from build123d import *

# Parameters (mm, degrees)
PAD_DEPTH           = 6
HOLE_D              = 6.6
HOLE_DEPTH          = 25
HOLE_CSINK_D        = 13.44
HOLE_CSINK_ANGLE    = 90
HOLE001_D           = 3.3
HOLE001_CSINK_D     = 4.05
HOLE001_CSINK_ANGLE = 90


with BuildPart() as part:
    # Sketch → Pad (new body)
    with BuildSketch(Plane.XY):
        with BuildLine():
            Line((0, 4.242641), (4.242641, 0))
            Line((177.999997, 0), (4.242641, 0))
            ThreePointArc((177.999997, 0), (179.414214, 0.585787), (180, 2.000004))
            Line((180, 161.757359), (180, 2.000004))
            Line((175.757359, 166), (180, 161.757359))
            Line((2.000009, 166), (175.757359, 166))
            ThreePointArc((2.000009, 166), (0.585793, 165.414221), (0, 164.000011))
            Line((0, 4.242641), (0, 164.000011))
        make_face()
    extrude(amount=PAD_DEPTH)

    # Hole
    with Locations(Plane.XY.offset(6)):
        with Locations((12, 154), (168, 154), (168, 12), (12, 12)):
            CounterSinkHole(HOLE_D / 2, HOLE_CSINK_D / 2, depth=HOLE_DEPTH, counter_sink_angle=HOLE_CSINK_ANGLE)

    # Hole001 (through all)
    with Locations(Plane.XY.offset(6)):
        with Locations((69.693453, 152.79207), (78.426115, 150.614773), (87.158776, 148.437476), (68, 146), (76.732662, 143.822703), (85.465323, 141.645406)):
            CounterSinkHole(HOLE001_D / 2, HOLE001_CSINK_D / 2, counter_sink_angle=HOLE001_CSINK_ANGLE)


solid = part.part
Geometry check sheet. Reference: the model listing, model coordinates, mm. Round coordinates to 2 decimals unless told otherwise and drop trailing zeros. Order: outer loops, then holes, each group sorted by start corner. A loop starts at its lowest first (then second) coordinate and runs counter-clockwise, first axis right, second up. Notation, with made-up numbers: (71, -40) - (91, -40) arc R27 cw to (91, -10) - close; hole circle Ø11 at (-4.75, 11.5). An arc over 180 degrees is marked (long way). One line per question, with ' | ' between items. Start each with the question number.
(1) Thickness scan on L1, parallel to Y at x = 168, z = 2.05; L2, parallel to X at y = 147, z = 1.65; L3, parallel to Y at x = 15, z = 5.1. Record the ranges inside material, lowest first. Write a range as [from, to].
(2) Sectioned sample at A-A on x = 12. Record the cut outline in (y, z), and give its area (3 significant figures).
(3) Sectioned sample at B-B on y = 12. Record the cut outline in (x, z).
(4) Depth check by flat-ended pin: pin 1 Ø6 at (x, y) = (12, 12) entering from -Z; pin 2 Ø8.5 at (x, y) = (168, 154) entering from +Z. Enter the tip coordinate at first touch or a pass-through.
(5) Release check for a two-part mould opening along Y. For faces 1 (the flat face through (89, 84, 0)), 2 (the conical face through (164.798, 10.672, 2.746)), 3 (the flat face through (92, 0, 3)) record: released by +Y, released by -Y, zero draft, split by the parting line, or undercut.
Conclusion:
1) L1: y = [0, 8.7], [15.3, 150.7], [157.3, 166] | L2: x = [0, 66.69], [69.31, 86.35], [87.97, 180] | L3: y = [0, 7.01], [16.99, 149.01], [158.99, 166]
2) outline: (0, 0) - (8.7, 0) - (8.7, 2.58) - (5.28, 6) - (0, 6) - close; (15.3, 0) - (150.7, 0) - (150.7, 2.58) - (147.28, 6) - (18.72, 6) - (15.3, 2.58) - close; (157.3, 0) - (166, 0) - (166, 6) - (160.72, 6) - (157.3, 2.58) - close | area: 893 mm2
3) outline: (0, 0) - (8.7, 0) - (8.7, 2.58) - (5.28, 6) - (0, 6) - close; (15.3, 0) - (164.7, 0) - (164.7, 2.58) - (161.28, 6) - (18.72, 6) - (15.3, 2.58) - close; (171.3, 0) - (180, 0) - (180, 6) - (174.72, 6) - (171.3, 2.58) - close
4) pin 1: passes through | pin 2: stops at z = 3.53
5) face 1: zero draft | face 2: undercut | face 3: released by -Y
